from build123d import *

# Parameters (mm, degrees)
SKETCH1_W           = 35
SKETCH1_H           = 20
BOSS_EXTRUDE1_DEPTH = 40
SKETCH2_R           = 12.7
CUT_EXTRUDE1_DEPTH  = 21
SKETCH3_R           = 1.75
CUT_EXTRUDE2_DEPTH  = 10


with BuildPart() as part:
    # Sketch1 → Boss-Extrude1 (new body)
    with BuildSketch(Plane(origin=(0, 0, 0), x_dir=(1, 0, 0), z_dir=(0, 1, 0))):
        with Locations((1.164675851, -0.855170824)):
            Rectangle(SKETCH1_W, SKETCH1_H)
    extrude(amount=BOSS_EXTRUDE1_DEPTH)

    # Sketch2 → Cut-Extrude1 (cut, through all)
    with BuildSketch(Plane.XY.offset(10.855170824)):
        with Locations((1.164675851, 25)):
            Circle(SKETCH2_R)
    extrude(amount=-CUT_EXTRUDE1_DEPTH, mode=Mode.SUBTRACT)

    # Sketch3 → Cut-Extrude2 (cut)
    with BuildSketch(Plane.XZ):
        with Locations((-8.335324149, 0.855170824)):
            Circle(SKETCH3_R)
        with Locations((10.664675851, 0.855170824)):
            Circle(SKETCH3_R)
    extrude(amount=-CUT_EXTRUDE2_DEPTH, mode=Mode.SUBTRACT)


solid = part.part
Model file for the job. Use its own axes, mm. A direction names the side the tool comes from. Round coordinates to 2 decimals unless told otherwise and drop trailing zeros. Loops run counter-clockwise (first coordinate to the right, second up) from the corner with the lowest first, then second, coordinate; pieces in that order, holes last.
1. Wall check: probe 1 along Y at (x, z) = (0, 8.5); probe 2 along Y at (x, z) = (10, 9.5); probe 3 along Z at (x, y) = (10, 6). Give the ranges that are in metal, low to high.
Check values:
probe 1: y = 0 to 12.35, 37.65 to 40
probe 2: y = 0 to 15.88, 34.12 to 40
probe 3: z = -9.14 to -0.76, 2.47 to 10.86
2. Band-saw the part on A-A, the plane y = 25. List the corners of the cut face in (x, z), and give its area (3 significant figures).
Check values:
outline: (-16.34, -9.14) - (-11.54, -9.14) - (-11.54, 10.86) - (-16.34, 10.86) - close; (13.86, -9.14) - (18.66, -9.14) - (18.66, 10.86) - (13.86, 10.86) - close
area: 192 mm2
3. Band-saw the part on B-B, the plane x = 4. List the corners of the cut face in (y, z), and give its area (3 significant figures).
Check values:
outline: (0, -9.14) - (12.62, -9.14) - (12.62, 10.86) - (0, 10.86) - close; (37.38, -9.14) - (40, -9.14) - (40, 10.86) - (37.38, 10.86) - close
area: 305 mm2
4. Tool access for faces 5 (the cylindrical face through (-10.084, 4.93, 0.932)), 6 (the flat face through (1, 0, 1)): list every direction of +Z, -Z, +X, -X, +Y, -Y with a clear straight run to the whole face (end or side of a thin tool).
Check values:
face 5: -Y
face 6: +Z, -Z, +X, -X, -Y
5. Band-saw the part on C-C, the plane z = -4.5. List the corners of the cut face in (x, y), and give its area (3 significant figures).
Check values:
outline: (-16.34, 0) - (18.66, 0) - (18.66, 40) - (-16.34, 40) - close; hole circle Ø25.4 at (1.16, 25)
area: 893 mm2
6. Band-saw the part on D-D, the plane z = 2. List the corners of the cut face in (x, y), and give its area (3 significant figures).
Check values:
outline: (-16.34, 0) - (-9.66, 0) - (-9.66, 10) - (-7.01, 10) - (-7.01, 0) - (9.34, 0) - (9.34, 10) - (11.99, 10) - (11.99, 0) - (18.66, 0) - (18.66, 40) - (-16.34, 40) - close; hole circle Ø25.4 at (1.16, 25)
area: 840 mm2
7. Mould opens along X. For faces 1 (the flat face through (1, 11, 10.855)), 2 (the flat face through (11, 10, 1)), 3 (the flat face through (-16.335, 20, 1)), 4 (the cylindrical face through (8.916, 4.93, 0.932)) say: +X half, -X half, draft (parallel to the pull), parting line (faces both ways), or undercut.
Check values:
face 1: draft
face 2: undercut
face 3: -X half
face 4: undercut
8. Drop a flat-ended pin along its axis: P1, Ø8, axis at x = -3.5, y = 32.5, coming from the -Z side. Give the stop position or say it passes through.
Check values:
P1: stops at z = -9.14
